Here's how the part is built. I have some questions about the finished solid (model axes, mm). Face numbers are marked on the shaded views. A direction names the side the tool comes from. Coordinates: 2 decimals unless noted, no trailing zeros. Order: outer loops, then holes, each group sorted by start corner. A loop starts at its lowest first (then second) coordinate and runs counter-clockwise, first axis right, second up. Notation, with made-up numbers: (55, -37) -> (86, -37) arc R11 cw to (86, -18) -> close; hole circle Ø4 at (41.25, 72.5). An arc over 180 degrees is marked (long way). One line per item, written item: value. Start each with the question number.
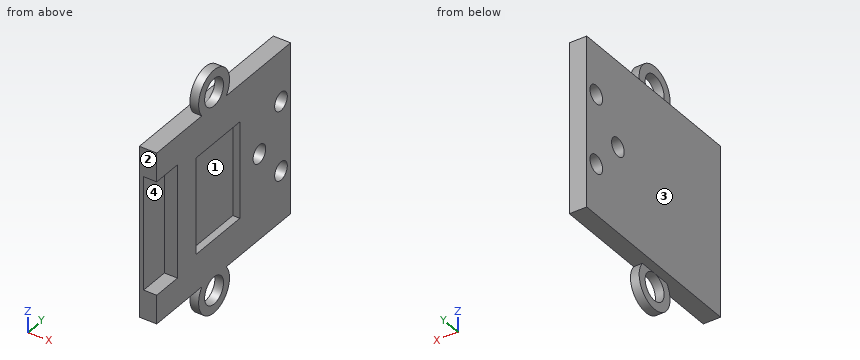
Autodesk Inventor part; units mm, degrees
ref_plane "YZ Plane" through (0, 0, 0) normal (1, 0, 0) x (0, 1, 0)
ref_plane "XZ Plane" through (0, 0, 0) normal (0, 1, 0) x (-1, 0, 0)
ref_plane "XY Plane" through (0, 0, 0) normal (0, 0, 1) x (1, 0, 0)
sketch "Sketch2" plane through (0, 0, 0) normal (1, 0, 0) x (0, 1, 0)
  line L0 (12, 15.675) -> (-12, 15.675)
  line L1 (-12, 15.675) -> (-12, -15.675)
  line L2 (-12, -15.675) -> (12, -15.675)
  line L3 (12, -15.675) -> (12, 15.675)
  point P0 (0, 0)
  dimension "d4" = 24
  dimension "d5" = 31.35
  dimension "d6" = 15.675
  dimension "d7" = 12
extrude "Extrusion1" add sketch "Sketch2" along normal blind 3.175
sketch "Sketch3" plane through (3.175, 0, 0) normal (1, 0, 0) x (0, 0, -1)
  line L0 (-15.675, -12) -> (15.675, -12)
  line L1 (-10.4, -12) -> (10.4, -12)
  line L2 (10.4, -12) -> (10.4, -6.5)
  line L3 (10.4, -6.5) -> (-10.4, -6.5)
  line L4 (-10.4, -6.5) -> (-10.4, -12)
  point P0 (0, 0)
  dimension "d16" = 20.8
  dimension "d17" = 10.4
  dimension "d18" = 5.5
extrude "Extrusion2" cut sketch "Sketch3" against normal blind 2.4
sketch "Sketch4" plane through (3.175, 0, 0) normal (1, 0, 0) x (0, 0, -1)
  line L0 (-8.85, 10) -> (8.85, 10)
  line L1 (8.85, 10) -> (8.85, -1.6)
  line L2 (8.85, -1.6) -> (-8.85, -1.6)
  line L3 (-8.85, -1.6) -> (-8.85, 10)
  line L4 (-10.4, -6.5) -> (10.4, -6.5)
  line L5 (10.4, -12) -> (-10.4, -12)
  point P0 (0, 4.2)
  dimension "d21" = 17.7
  dimension "d22" = 8.85
  dimension "d23" = 5.8
  dimension "d24" = 11.6
  dimension "d27" = 10.4
extrude "Extrusion3" cut sketch "Sketch4" against normal blind 1.3
sketch "Sketch5" plane through (3.175, 0, 0) normal (1, 0, 0) x (0, 0, -1)
  circle A0 centre (-10.65, 10.9) radius 0.8411
  circle A1 centre (10.65, 10.9) radius 0.8411
  line L0 (-15.675, 12) -> (-15.675, -12)
  line L1 (15.675, 12) -> (-15.675, 12)
  line L2 (15.675, -12) -> (15.675, 12)
  line L3 (8.85, 10) -> (8.85, -1.6)
  line L4 (-8.85, 10) -> (8.85, 10)
  point P0 (0, 0)
  dimension "d31" = 1.6822
  dimension "d33" = 1.6822
  dimension "d60" = 1.8
  dimension "d62" = 0.9
  dimension "d67" = 0.9
  dimension "d68" = 1.8
extrude "Extrusion7" [suppressed]
sketch "Sketch10" plane through (3.175, 0, 0) normal (1, 0, 0) x (0, 0, -1)
  circle A0 centre (-18.175, 3.175) radius 2.5
  line L0 (-15.675, 12) -> (-15.675, -12) construction
  arc A1 (-15.675, 6.4088) -> (-15.675, -0.0588) centre (-18.175, 3.175) ccw
  line L1 (0, 13.5875) -> (0, -23.7475) construction
  circle A2 centre (18.175, 3.175) radius 2.5
  arc A3 (15.675, -0.0588) -> (15.675, 6.4088) centre (18.175, 3.175) ccw
  line L2 (15.675, 12) -> (-15.675, 12)
  line L3 (-15.675, 6.4088) -> (-15.675, -0.0588)
  line L4 (15.675, -12) -> (15.675, 12)
  line L5 (15.675, 6.4088) -> (15.675, -0.0588)
  point P0 (0, 0)
  dimension "d73" = 8.175
  dimension "d74" = 5
  dimension "d80" = 24
  dimension "d81" = 15.175
extrude "Extrusion13" add sketch "Sketch10" against normal blind 1.5875
sketch "Sketch12" plane through (0, 12, 15.675) normal (0, 1, 0) x (1, 0, 0)
  line L0 (0, 31.35) -> (0, 0)
  line L1 (0, 0) -> (3.175, 0)
  line L2 (3.175, 31.35) -> (3.175, 0)
  line L3 (0, 31.35) -> (3.175, 31.35)
  point P0 (0, 15.675)
extrude "Extrusion14" add sketch "Sketch12" along normal blind 11.43
sketch "Sketch13" plane through (0, 0, 0) normal (-1, 0, 0) x (0, 0, 1)
  circle A0 centre (-6.3786, 20.89) radius 1.6764
  circle A1 centre (6.3786, 20.89) radius 1.6764
  line L0 (-15.675, 23.43) -> (15.675, 23.43)
  line L1 (-15.675, -12) -> (-15.675, 23.43)
  line L2 (15.675, 23.43) -> (15.675, -12)
  circle A2 centre (0, 15.175) radius 1.6764
  point P0 (0, 0)
  dimension "d92" = 3.3528
  dimension "d93" = 3.3528
  dimension "d94" = 2.54
  dimension "d95" = 9.2964
  dimension "d96" = 9.2964
  dimension "d97" = 2.54
  dimension "d98" = 3.3528
  dimension "d99" = 8.255
  dimension "d100" = 31.35
  dimension "d101" = 15.675
extrude "Extrusion15" cut sketch "Sketch13" against normal through all
equation "\"d31\" = d30"
equation "\"d33\" = d30"
equation "\"d67\" = d62"
equation "\"d68\" = d60"
equation "\"d93\" = d92"
equation "\"d96\" = d95"
equation "\"d98\" = d92"
equation "\"d101\" = 0.5 * d100"
properties part number "Pi cCam Mount" material "Aluminum 6061-AHC"
Q1. I need wall thicknesses on line 1 (Z direction, x = 2.65, y = 3); line 2 (Z direction, x = 3.05, y = 15) (3 decimals); line 3 (Y direction, x = 1.95, z = 6). Which ranges of each line are inside material? Lowest first, please.
Q2. Imagine slicing it at B-B (y = 20.89). Write out the boundary of the cut face in (x, z) (3 decimals), plus the area to 3 significant figures.
Q3. For the marked faces 3 and 4, which set-ups out of +Z, -Z, +X, -X, +Y, -Y let a thin tool reach every point of the face, with its end or its side?
Q4. Imagine slicing it at A-A (z = 0). Write out the boundary of the cut face in (x, y) (3 decimals).
Q5. For P1, Ø4, axis at y = 3.175, z = -18.175, coming from the -X side; P2, Ø1.2, axis at x = 2, y = -10, coming from the -Z side (3 decimals); P3, Ø1, axis at x = 2.5, y = 2, coming from the +Z side; P4, Ø1.9, axis at x = 2, y = -10, coming from the +Z side (3 decimals), each with a flat end and sliding along its axis, tell me the tip position at first contact or that it passes through.
Q6. Imagine slicing it at C-C (z = 18.5). Write out the boundary of the cut face in (x, y) (1 decimal).
Q7. If we mould it in two halves opening along Z, with no side actions, what happens to the marked faces 1 and 2? For each: +Z half, -Z half, draft (parallel to the pull), parting line (faces both ways), or undercut.
Q8. Imagine slicing it at D-D (y = -5.5). Write out the boundary of the cut face in (x, z) (3 decimals).
Completed:
1. line 1: z = -22.26 to -20.67, -15.68 to -8.85, 8.85 to 15.68, 20.67 to 22.26
1. line 2: z = -15.675 to -1.667, 1.667 to 15.675
1. line 3: y = -6.5 to -1.6, 10 to 19.26, 22.52 to 23.43
2. outline: (0, -15.675) -> (3.175, -15.675) -> (3.175, -8.055) -> (0, -8.055) -> close; (0, -4.702) -> (3.175, -4.702) -> (3.175, 4.702) -> (0, 4.702) -> close; (0, 8.055) -> (3.175, 8.055) -> (3.175, 15.675) -> (0, 15.675) -> close
2. area: 78.2 mm2
3. face 3: +Z, -Z, -X, +Y, -Y
3. face 4: +X, -Y
4. outline: (0, -12) -> (0.775, -12) -> (0.775, -6.5) -> (3.175, -6.5) -> (3.175, -1.6) -> (1.875, -1.6) -> (1.875, 10) -> (3.175, 10) -> (3.175, 13.499) -> (0, 13.499) -> close; (0, 16.851) -> (3.175, 16.851) -> (3.175, 23.43) -> (0, 23.43) -> close
5. P1: passes through
5. P2: stops at z = -15.675
5. P3: stops at z = 22.21
5. P4: stops at z = 15.675
6. outline: (1.6, -0.9) -> (3.2, -0.9) -> (3.2, 0.7) -> (1.6, 0.7) -> close; (1.6, 5.7) -> (3.2, 5.7) -> (3.2, 7.2) -> (1.6, 7.2) -> close
7. face 1: undercut
7. face 2: draft
8. outline: (0, -15.675) -> (3.175, -15.675) -> (3.175, 15.675) -> (0, 15.675) -> close
